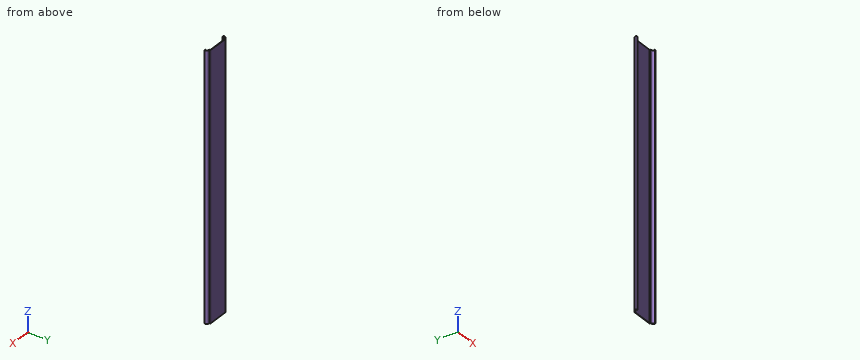
from build123d import *

# Parameters (mm, degrees)
EXTRUDE_THIN1_DEPTH = 825.5
FILLET1_R           = 1.27


with BuildPart() as part:
    # Sketch1 → Extrude-Thin1 (new body)
    with BuildSketch(Plane.XY):
        with BuildLine():
            Line((-38.1, 0), (-41.275, 0))
            ThreePointArc((-41.275, 0), (-39.354822583, 7.228599878), (-32.54375, 10.31875))
            Line((-32.54375, 10.31875), (-32.54375, 12.7))
            Line((-32.54375, 12.7), (32.54375, 12.7))
            Line((32.54375, 12.7), (32.54375, 10.31875))
            ThreePointArc((32.54375, 10.31875), (39.354822583, 7.228599878), (41.275, 0))
            Line((41.275, 0), (38.1, 0))
            Line((38.1, 0), (38.1, 1.27))
            Line((38.1, 1.27), (40.143945779, 1.27))
            ThreePointArc((40.143945779, 1.27), (37.560409803, 7.240667538), (31.27375, 8.914417078))
            Line((31.27375, 8.914417078), (31.27375, 11.43))
            Line((31.27375, 11.43), (-31.27375, 11.43))
            Line((-31.27375, 11.43), (-31.27375, 8.914417078))
            ThreePointArc((-31.27375, 8.914417078), (-37.560409803, 7.240667538), (-40.143945779, 1.27))
            Line((-40.143945779, 1.27), (-38.1, 1.27))
            Line((-38.1, 1.27), (-38.1, 0))
        make_face()
    extrude(amount=-EXTRUDE_THIN1_DEPTH)

    # Fillet1
    fillet1_edges = [part.edges().sort_by_distance(p)[0] for p in [
        (-41.275, 0, -412.75),
        (-32.54375, 12.7, -412.75),
        (32.54375, 12.7, -412.75),
        (41.275, 0, -412.75),
        (31.27375, 8.914417078, -412.75),
        (-31.27375, 8.914417078, -412.75),
    ]]
    fillet(fillet1_edges, radius=FILLET1_R)


solid = part.part
Geometry: final body of the model. Coordinates: model frame, mm. Coordinates: 2 decimals unless noted, no trailing zeros. Loops run counter-clockwise (first coordinate to the right, second up) from the corner with the lowest first, then second, coordinate; pieces in that order, holes last. Notation, with made-up numbers: (-1.75, 78.5) - (11.25, 78.5) arc R12 ccw to (11.25, 87.5) - close; hole circle Ø9 at (6.25, -29.5). An arc over 180 degrees is marked (long way). One line per question, with ' | ' between items. Start each with the question number.
(1) Ray query, L1, parallel to X at y = 11.25, z = -649.5; L2, parallel to X at y = 2.5, z = -202; L3, parallel to Y at x = 8.5, z = -346. Return the intervals inside material, ascending. Write a range as from..to.
(2) Cut plane A-A on y = 3.25. Output: boundary loops of the cut face in (x, z).
(3) Cut plane B-B on z = -286. Output: boundary loops of the cut face in (x, y).
(4) First-contact query: pin 1 (0.9 mm diameter, centred on y = 11, z = -331.5, fed in from -X); pin 2 (2 mm diameter, centred on y = 5.5, z = -442, fed in from +X); pin 3 (1 mm diameter, centred on x = 38.5, z = -286, fed in from +Y); pin 4 (1 mm diameter, centred on x = -1.5, y = 9.5, fed in from +Z). Flat tips, straight axial feed; report the tip coordinate or a pass-through.
(5) Cut plane C-C on x = -18. Output: boundary loops of the cut face in (y, z), and give its area (3 significant figures).
Here are the results:
1) L1: -32.54..-31.27, 31.27..32.54 | L2: -41.37..-40.09, 40.09..41.37 | L3: 11.43..12.7
2) outline: (-41.26, -825.5) - (-39.96, -825.5) - (-39.96, 0) - (-41.26, 0) - close; (39.96, -825.5) - (41.26, -825.5) - (41.26, 0) - (39.96, 0) - close
3) outline: (-41.41, 1.22) arc R1.27 ccw to (-40.14, 0) - (-38.1, 0) - (-38.1, 1.27) - (-40.14, 1.27) arc R7.46 cw to (-32.56, 9.05) arc R1.27 ccw to (-31.27, 10.32) - (-31.27, 11.43) - (31.27, 11.43) - (31.27, 10.32) arc R1.27 ccw to (32.56, 9.05) arc R7.46 cw to (40.14, 1.27) - (38.1, 1.27) - (38.1, 0) - (40.14, 0) arc R1.27 ccw to (41.41, 1.22) arc R8.73 ccw to (32.54, 10.32) - (32.54, 11.43) arc R1.27 ccw to (31.27, 12.7) - (-31.27, 12.7) arc R1.27 ccw to (-32.54, 11.43) - (-32.54, 10.32) arc R8.73 ccw to start
4) pin 1: x = -32.54 | pin 2: x = 40.92 | pin 3: y = 8.52 | pin 4: through
5) outline: (11.43, -825.5) - (12.7, -825.5) - (12.7, 0) - (11.43, 0) - close | area: 1,050 mm²
